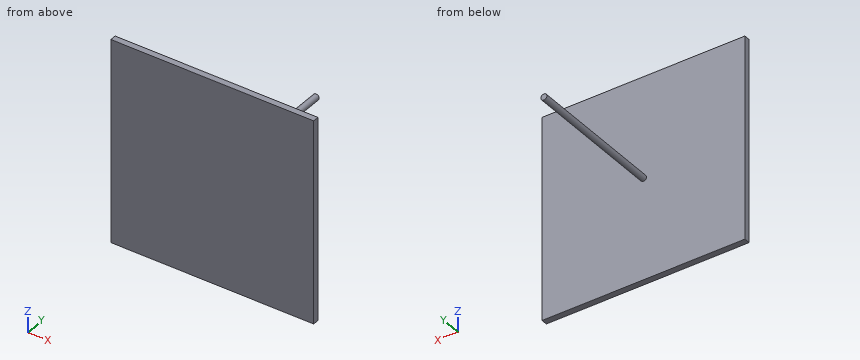
from build123d import *

# Parameters (mm, degrees)
ESTRUSIONE_ESTRUSIONE1_START = 70
SCHIZZO1_W                   = 100
SCHIZZO1_H                   = 100
ESTRUSIONE_ESTRUSIONE1_DEPTH = 3
SCHIZZO2_R                   = 1.5
ESTRUSIONE_ESTRUSIONE2_DEPTH = 70


with BuildPart() as part:
    # Schizzo1 → Estrusione-Estrusione1 (new body)
    with BuildSketch(Plane.XZ.offset(24.14).offset(ESTRUSIONE_ESTRUSIONE1_START)):
        with Locations((-167.062548693, -37.708245302)):
            Rectangle(SCHIZZO1_W, SCHIZZO1_H)
    extrude(amount=ESTRUSIONE_ESTRUSIONE1_DEPTH)

    # Schizzo2 → Estrusione-Estrusione2 (add)
    with BuildSketch(Plane(origin=(0, -94.14, 0), x_dir=(1, 0, 0), z_dir=(0, 1, 0))):
        with Locations((-167.062548693, 37.708245302)):
            Circle(SCHIZZO2_R)
    extrude(amount=ESTRUSIONE_ESTRUSIONE2_DEPTH)


solid = part.part
Design review of the part built by this model. Coordinates are the model's own, in mm. Round coordinates to 2 decimals unless told otherwise and drop trailing zeros. Write each loop counter-clockwise with the first axis right and the second up, starting at its lowest first coordinate (ties: lowest second). Pieces come first, ordered by that corner, then holes. Notation, with made-up numbers: (28, 18.25) -> (81, 18.25) arc R9 cw to (81, 26.25) -> close; hole circle Ø8 at (36, 36). An arc over 180 degrees is marked (long way). One line per item, written item: value. Start each with the question number.
Q1. Add section B-B (z = -60). Give the boundary of the cut face in (x, y), then the cut area to 3 significant figures.
Q2. To check wall thickness, follow probe 1 along Y at (x, z) = (-198, -1.5); probe 2 along X at (y, z) = (-66.5, -37). State the ranges of each line that lie inside material, in increasing order.
Q3. Add section A-A (x = -144). Give the boundary of the cut face in (y, z).
Q4. Add section C-C (y = -79). Give the boundary of the cut face in (x, z), then the cut area to 3 significant figures.
Q5. Insertion check: P1, Ø1.5, axis at x = -156, z = -51, coming from the +Y side; P2, Ø10, axis at y = -52, z = -27.5, coming from the -X side. Each pin has a flat end and moves straight along its axis. Give the tip position at first contact, or say it passes through.
Response:
1. outline: (-217.06, -97.14) -> (-117.06, -97.14) -> (-117.06, -94.14) -> (-217.06, -94.14) -> close
1. area: 300 mm^2
2. probe 1: y = -97.14 to -94.14
2. probe 2: x = -168.38 to -165.74
3. outline: (-97.14, -87.71) -> (-94.14, -87.71) -> (-94.14, 12.29) -> (-97.14, 12.29) -> close
4. outline: circle Ø3 at (-167.06, -37.71)
4. area: 7.07 mm^2
5. P1: stops at y = -94.14
5. P2: passes through
